Input: part model. Units: mm. Frame: model coordinates. A direction names the side the tool comes from. Round coordinates to 2 decimals unless told otherwise and drop trailing zeros. Loops run counter-clockwise (first coordinate to the right, second up) from the corner with the lowest first, then second, coordinate; pieces in that order, holes last. Notation, with made-up numbers: (22.5, 84) -> (64.5, 84) arc R25 cw to (64.5, 110) -> close; hole circle Ø9 at (10, 8). An arc over 180 degrees is marked (long way). Answer as a JSON object with one key per item and string values.
```python
from build123d import *

# Parameters (mm, degrees)
F0_R     = 2.54
F1_DEPTH = 7.62
F2_DEPTH = 15.24
F3_DEPTH = 20.32


with BuildPart() as f1:
    # F0 (on Front) → F1 (new body)
    with BuildSketch(Plane.XZ):
        with BuildLine():
            ThreePointArc((-8.7988181024, -5.08), (-9.8138063951, -2.6296014982), (-10.16, 0))
            ThreePointArc((-10.16, 0), (-9.8138063951, 2.6296014982), (-8.7988181024, 5.08))
            Line((-8.7988181024, 5.08), (-25.4, 5.08))
            ThreePointArc((-25.4, 5.08), (-30.48, 0), (-25.4, -5.08))
            Line((-25.4, -5.08), (-8.7988181024, -5.08))
        make_face()
        with Locations((-25.4, 0)):
            Circle(F0_R, mode=Mode.SUBTRACT)
        with Locations((-25.4, 0)):
            Circle(F0_R)
        with BuildLine():
            Line((-10.16, 0), (10.16, 0))
            ThreePointArc((10.16, 0), (9.8138063951, 2.6296014982), (8.7988181025, 5.08))
            Line((8.7988181025, 5.08), (-8.7988181024, 5.08))
            ThreePointArc((-8.7988181024, 5.08), (-9.8138063951, 2.6296014982), (-10.16, 0))
        make_face()
        with BuildLine():
            ThreePointArc((8.7988181025, -5.08), (9.8138063951, -2.6296014982), (10.16, 0))
            Line((10.16, 0), (-10.16, 0))
            ThreePointArc((-10.16, 0), (-9.8138063951, -2.6296014982), (-8.7988181024, -5.08))
            Line((-8.7988181024, -5.08), (8.7988181025, -5.08))
        make_face()
        with BuildLine():
            ThreePointArc((8.7988181025, 5.08), (9.8138063951, 2.6296014982), (10.16, 0))
            ThreePointArc((10.16, 0), (9.8138063951, -2.6296014982), (8.7988181025, -5.08))
            Line((8.7988181025, -5.08), (25.4, -5.08))
            ThreePointArc((25.4, -5.08), (30.48, 0), (25.4, 5.08))
            Line((25.4, 5.08), (8.7988181025, 5.08))
        make_face()
        with BuildLine():
            ThreePointArc((27.94, 0), (25.4, -2.54), (22.86, 0))
            ThreePointArc((22.86, 0), (25.4, 2.54), (27.94, 0))
        make_face(mode=Mode.SUBTRACT)
        with BuildLine():
            ThreePointArc((27.94, 0), (25.4, 2.54), (22.86, 0))
            ThreePointArc((22.86, 0), (25.4, -2.54), (27.94, 0))
        make_face()
        with BuildLine():
            Line((-8.7988181024, 5.08), (8.7988181025, 5.08))
            ThreePointArc((8.7988181025, 5.08), (0, 10.16), (-8.7988181024, 5.08))
        make_face()
        with BuildLine():
            ThreePointArc((-8.7988181024, -5.08), (0, -10.16), (8.7988181025, -5.08))
            Line((8.7988181025, -5.08), (-8.7988181024, -5.08))
        make_face()
    extrude(amount=F1_DEPTH)

    # F0 (on Front) → F2 (join)
    with BuildSketch(Plane.XZ):
        with BuildLine():
            Line((-8.7988181024, 5.08), (8.7988181025, 5.08))
            ThreePointArc((8.7988181025, 5.08), (0, 10.16), (-8.7988181024, 5.08))
        make_face()
        with BuildLine():
            Line((-10.16, 0), (10.16, 0))
            ThreePointArc((10.16, 0), (9.8138063951, 2.6296014982), (8.7988181025, 5.08))
            Line((8.7988181025, 5.08), (-8.7988181024, 5.08))
            ThreePointArc((-8.7988181024, 5.08), (-9.8138063951, 2.6296014982), (-10.16, 0))
        make_face()
        with BuildLine():
            ThreePointArc((8.7988181025, -5.08), (9.8138063951, -2.6296014982), (10.16, 0))
            Line((10.16, 0), (-10.16, 0))
            ThreePointArc((-10.16, 0), (-9.8138063951, -2.6296014982), (-8.7988181024, -5.08))
            Line((-8.7988181024, -5.08), (8.7988181025, -5.08))
        make_face()
        with BuildLine():
            ThreePointArc((-8.7988181024, -5.08), (0, -10.16), (8.7988181025, -5.08))
            Line((8.7988181025, -5.08), (-8.7988181024, -5.08))
        make_face()
    extrude(amount=F2_DEPTH)

    # F0 (on Front) → F3 (join)
    with BuildSketch(Plane.XZ):
        with Locations((-25.4, 0)):
            Circle(F0_R)
        with BuildLine():
            ThreePointArc((27.94, 0), (25.4, 2.54), (22.86, 0))
            ThreePointArc((22.86, 0), (25.4, -2.54), (27.94, 0))
        make_face()
    extrude(amount=F3_DEPTH)


solid = f1.part
```
1) Reachability of faces 4 (the face through (-27.938, -13.881, 0.112)), 5 (the face through (17, -4, -5.08)), 6 (the face through (-17, -4, 5.08)) from +Z, -Z, +X, -X, +Y, -Y: full face, straight path, thin tool, end or side. Return the list, or none.
Output:
{"face 4": "-Y", "face 5": "-Z, +X, +Y, -Y", "face 6": "+Z, -X, +Y, -Y"}
2) Section A-A, the plane z = 0. Output: boundary loops of the cut face in (x, y).
Output:
{"outline": "(-30.48, -7.62) -> (-27.94, -7.62) -> (-27.94, -20.32) -> (-22.86, -20.32) -> (-22.86, -7.62) -> (-10.16, -7.62) -> (-10.16, -15.24) -> (10.16, -15.24) -> (10.16, -7.62) -> (22.86, -7.62) -> (22.86, -20.32) -> (27.94, -20.32) -> (27.94, -7.62) -> (30.48, -7.62) -> (30.48, 0) -> (-30.48, 0) -> close"}
3) Contact query for flat-ended pins moving along their axis: P1, Ø2.5, axis at x = 18.5, y = -5.5, coming from the -Z side; P2, Ø4, axis at x = 16, y = -5, coming from the +Z side; P3, Ø10, axis at x = 0, z = -0.5, coming from the -Y side. Output: stop coordinate, or through.
Output:
{"P1": "stops at z = -5.08", "P2": "stops at z = 5.08", "P3": "stops at y = -15.24"}
4) Draft query along X for faces 1 (the face through (19, -7.62, 0)), 2 (the face through (30.48, -3.76, -0.11)), 3 (the face through (17, -4, 5.08)). Return one class per face: +X half, -X half, draft (parallel to the pull), parting line (faces both ways), or undercut.
Output:
{"face 1": "undercut", "face 2": "+X half", "face 3": "draft"}
5) Section D-D, the plane x = -14.5. Output: boundary loops of the cut face in (y, z), plus the area to 3 significant figures.
Output:
{"outline": "(-7.62, -5.08) -> (0, -5.08) -> (0, 5.08) -> (-7.62, 5.08) -> close", "area": "77.4 mm^2"}
6) Section B-B, the plane y = -13.75. Output: boundary loops of the cut face in (x, z), plus the area to 3 significant figures.
Output:
{"outline": "circle Ø5.08 at (-25.4, 0); circle Ø20.32 at (0, 0); circle Ø5.08 at (25.4, 0)", "area": "365 mm^2"}
7) Section C-C, the plane y = -5.75. Output: boundary loops of the cut face in (x, z).
Output:
{"outline": "(-25.4, -5.08) -> (-8.8, -5.08) arc R10.16 ccw to (8.8, -5.08) -> (25.4, -5.08) arc R5.08 ccw to (25.4, 5.08) -> (8.8, 5.08) arc R10.16 ccw to (-8.8, 5.08) -> (-25.4, 5.08) arc R5.08 ccw to start"}
8) Ray query, probe 1 along Y at (x, z) = (-8, -0.25); probe 2 along X at (y, z) = (-12.5, -1); probe 3 along Y at (x, z) = (-22, -2.25). Return the intervals inside material, ascending.
Output:
{"probe 1": "y = -15.24 to 0", "probe 2": "x = -27.73 to -23.07, -10.11 to 10.11, 23.07 to 27.73", "probe 3": "y = -7.62 to 0"}
